from build123d import *

# Parameters (mm, degrees)
F1_DEPTH = 40.2336
F0_R     = 10.16
F2_DEPTH = 15.7734
F3_R     = 1.27


with BuildPart() as f1:
    # F0 (on Top) → F1 (new body)
    with BuildSketch(Plane.XY):
        with BuildLine():
            ThreePointArc((5.042647, -28.126541), (21.916025, -18.336262), (28.575, 0))
            ThreePointArc((28.575, 0), (21.916025, 18.336262), (5.042647, 28.126541))
            ThreePointArc((5.042647, 28.126541), (-28.575, 0), (5.042647, -28.126541))
        make_face()
        with BuildLine():
            ThreePointArc((15.788915, -4.826), (-16.51, 0), (15.788915, 4.826))
            Line((15.788915, 4.826), (24.240017, 4.826))
            Line((24.240017, 4.826), (24.240017, -4.826))
            Line((24.240017, -4.826), (15.788915, -4.826))
        make_face(mode=Mode.SUBTRACT)
    extrude(amount=F1_DEPTH)

    # F0 (on Top) → F2 (join)
    with BuildSketch(Plane.XY):
        with BuildLine():
            ThreePointArc((73.025, 0), (68.585683, 12.224174), (57.336765, 18.751028))
            ThreePointArc((57.336765, 18.751028), (34.925, 0), (57.336765, -18.751028))
            ThreePointArc((57.336765, -18.751028), (68.585683, -12.224174), (73.025, 0))
        make_face()
        with Locations((53.975, 0)):
            Circle(F0_R, mode=Mode.SUBTRACT)
        with BuildLine():
            ThreePointArc((5.042647, 28.126541), (21.916025, 18.336262), (28.575, 0))
            ThreePointArc((28.575, 0), (21.916025, -18.336262), (5.042647, -28.126541))
            Line((5.042647, -28.126541), (57.336765, -18.751028))
            ThreePointArc((57.336765, -18.751028), (34.925, 0), (57.336765, 18.751028))
            Line((57.336765, 18.751028), (5.042647, 28.126541))
        make_face()
    extrude(amount=F2_DEPTH)

    # F3
    f3_edges = [f1.edges().sort_by_distance(p)[0] for p in [
        (-5.042647, 28.126541, 40.2336),
    ]]
    fillet(f3_edges, radius=F3_R)


solid = f1.part
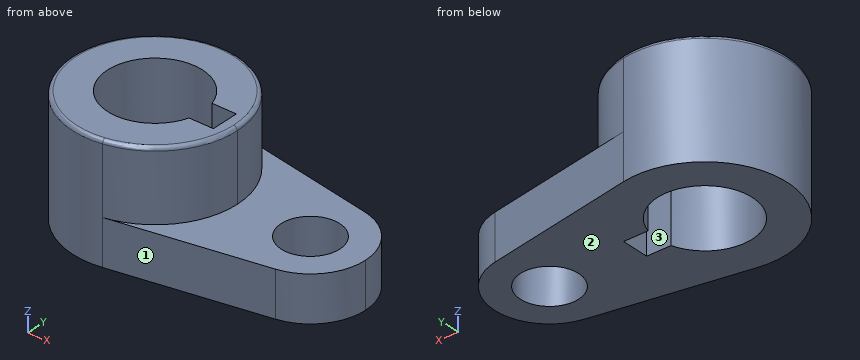
Design review of the part built by this model. Coordinates are the model's own, in mm. Face numbers are marked on the shaded views. Coordinates: 2 decimals unless noted, no trailing zeros. Order: outer loops, then holes, each group sorted by start corner. A loop starts at its lowest first (then second) coordinate and runs counter-clockwise, first axis right, second up. Notation, with made-up numbers: (43.25, -32) -> (84.25, -32) arc R24 cw to (84.25, 7) -> close; hole circle Ø9 at (2, 49.5). An arc over 180 degrees is marked (long way). One line per item, written item: value.
1) Draft analysis for pull direction Y (two halves, no side actions). For the marked faces 1, 2 and 3, state which applies: +Y half, -Y half, draft (parallel to the pull), parting line (faces both ways), or undercut.
Output values:
face 1: -Y half
face 2: draft
face 3: undercut
2) We need section A-A, the plane z = 34. Give the boundary of the cut face in (x, y) (3 decimals).
Output values:
outline: (5.043, -28.127) arc R28.575 ccw to (28.575, 0) arc R28.575 ccw to (5.043, 28.127) arc R28.575 ccw (long way) to start; hole (15.789, -4.826) -> (24.24, -4.826) -> (24.24, 4.826) -> (15.789, 4.826) arc R16.51 ccw (long way) to start
3) We need section C-C, the plane x = 49.5. Give the boundary of the cut face in (y, z).
Output values:
outline: (-20.16, 0) -> (-9.12, 0) -> (-9.12, 15.77) -> (-20.16, 15.77) -> close; (9.12, 0) -> (20.16, 0) -> (20.16, 15.77) -> (9.12, 15.77) -> close
4) Clearance check with flat-ended pins moving along their axes: P1, Ø8, axis at x = 49.5, z = 17, coming from the -Y side; P2, Ø7.5, axis at y = -0.5, z = 17.5, coming from the -X side (3 decimals); P3, Ø5, axis at x = 59.5, y = -10.5, coming from the +Z side. State where each tip first meets the part, or that it passes through.
Output values:
P1: stops at y = -20.84
P2: stops at x = -28.575
P3: stops at z = 15.77
5) We need section B-B, the plane z = 6. Give the boundary of the cut face in (x, y) (3 decimals), then the cut area to 3 significant figures.
Output values:
outline: (5.043, -28.127) -> (57.337, -18.751) arc R19.05 ccw to (73.025, 0) arc R19.05 ccw to (57.337, 18.751) -> (5.043, 28.127) arc R28.575 ccw (long way) to start; hole (15.789, -4.826) -> (24.24, -4.826) -> (24.24, 4.826) -> (15.789, 4.826) arc R16.51 ccw (long way) to start; hole circle Ø20.32 at (53.975, 0)
area: 3,210 mm2
6) To check wall thickness, follow probe 1 along Y at (x, z) = (0, 23) (3 decimals); probe 2 along Z at (x, y) = (49.5, -17.5); probe 3 along Y at (x, z) = (62, 15.5). State the ranges of each line that lie inside material, in increasing order. Write a range as [from, to].
Output values:
probe 1: y = [-28.575, -16.51], [16.51, 28.575]
probe 2: z = [0, 15.77]
probe 3: y = [-17.28, -6.23], [6.23, 17.28]
